Source: CAD feature listing. Evaluate the final solid. Frame: model axes, mm. Face numbers are marked on the shaded views. A direction names the side the tool comes from. Give positions to 0.01 mm unless a question says otherwise; leave off trailing zeros. Write each loop counter-clockwise with the first axis right and the second up, starting at its lowest first coordinate (ties: lowest second). Pieces come first, ordered by that corner, then holes. Notation, with made-up numbers: (82, 76) -> (91, 76) arc R16 ccw to (91, 80) -> close; hole circle Ø9 at (76.5, 62). An arc over 180 degrees is marked (long way). Answer as a JSON object with one key per item and string values. Group by question number.
Item 1: Access query for the marked faces 1, 2 and 3. Directions: +Z, -Z, +X, -X, +Y, -Y. A direction counts if a zero-diameter tool reaches every point of the face in a straight line with its end or side. Return the directions, or none.
Item 2: Section query B-B on z = 0.75. Return the cut outline in (x, y).
Item 3: Section query D-D on x = 21.5. Return the cut outline in (y, z), plus the area to 3 significant figures.
Item 4: First-contact query: pin 1 Ø1 at (x, z) = (7, 1.5) entering from -Y; pin 2 Ø1.2 at (y, z) = (3.5, 1) entering from -X; pin 3 Ø2.5 at (x, y) = (8, 0) entering from +Z. Flat tips, straight axial feed; report the tip coordinate or a pass-through.
Item 5: Ray query, probe 1 along X at (y, z) = (-1.5, 0.6); probe 2 along Z at (x, y) = (22, 1); probe 3 along Y at (x, z) = (2, 0.85). Return the intervals inside material, ascending. Write a range as from..to.
Item 6: Section query A-A on x = 4. Return the cut outline in (y, z), plus the area to 3 significant figures.
Item 7: Section query C-C on y = 0. Return the cut outline in (x, z), plus the area to 3 significant figures.
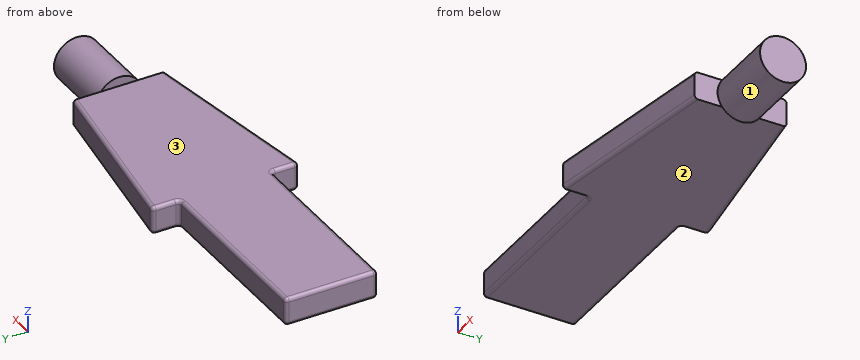
from build123d import *

# Parameters (mm, degrees)
F1_DEPTH = 1.5
F2_R     = 1.25
F3_DEPTH = 4
F4_R     = 0.2


with BuildPart() as f1:
    # F0 (on Top) → F1 (new body)
    with BuildSketch(Plane.XY):
        Polygon((0, 2.5), (0, 0), (0, -2.5), (10, -2.5), (10, -4), (20, -2.5), (20, 0), (20, 2.5), (10, 4), (10, 2.5), align=None)
    extrude(amount=F1_DEPTH)

    # F2 (on face) → F3 (join)
    with BuildSketch(Plane.YZ.offset(20)):
        with Locations((0, 0.75)):
            Circle(F2_R)
    extrude(amount=F3_DEPTH)

    # F4
    f4_edges = [f1.edges().sort_by_distance(p)[0] for p in [
        (5, -2.5, 1.5),
        (0, 0, 1.5),
        (5, 2.5, 1.5),
        (15, 3.25, 1.5),
        (15, -3.25, 1.5),
        (10, -3.25, 1.5),
        (10, 3.25, 1.5),
        (10, -3.25, 0),
        (15, -3.25, 0),
        (5, -2.5, 0),
        (0, 0, 0),
        (10, 3.25, 0),
        (5, 2.5, 0),
        (15, 3.25, 0),
        (10, 4, 0.75),
        (10, 2.5, 0.75),
        (10, -2.5, 0.75),
        (10, -4, 0.75),
        (0, -2.5, 0.75),
        (0, 2.5, 0.75),
    ]]
    fillet(f4_edges, radius=F4_R)


solid = f1.part
Worked answers:
{
 "1": {"face 1": "+X", "face 2": "-Z, -X, +Y, -Y", "face 3": "+Z, -X, +Y, -Y"},
 "2": {"outline": "(0, -2.3) arc R0.2 ccw to (0.2, -2.5) -> (9.8, -2.5) arc R0.2 cw to (10, -2.7) -> (10, -3.77) arc R0.2 ccw to (10.23, -3.97) -> (20, -2.5) -> (20, -1.25) -> (24, -1.25) -> (24, 1.25) -> (20, 1.25) -> (20, 2.5) -> (10.23, 3.97) arc R0.2 ccw to (10, 3.77) -> (10, 2.7) arc R0.2 cw to (9.8, 2.5) -> (0.2, 2.5) arc R0.2 ccw to (0, 2.3) -> close"},
 "3": {"outline": "circle Ø2.5 at (0, 0.75)", "area": "4.91 mm^2"},
 "4": {"pin 1": "y = -2.5", "pin 2": "x = 10", "pin 3": "z = 1.5"},
 "5": {"probe 1": "0..20", "probe 2": "0..1.5", "probe 3": "-2.5..2.5"},
 "6": {"outline": "(-2.5, 0.2) arc R0.2 ccw to (-2.3, 0) -> (2.3, 0) arc R0.2 ccw to (2.5, 0.2) -> (2.5, 1.3) arc R0.2 ccw to (2.3, 1.5) -> (-2.3, 1.5) arc R0.2 ccw to (-2.5, 1.3) -> close", "area": "7.47 mm^2"},
 "7": {"outline": "(0, 0.2) arc R0.2 ccw to (0.2, 0) -> (20, 0) -> (20, -0.5) -> (24, -0.5) -> (24, 2) -> (20, 2) -> (20, 1.5) -> (0.2, 1.5) arc R0.2 ccw to (0, 1.3) -> close", "area": "40.0 mm^2"}
}
